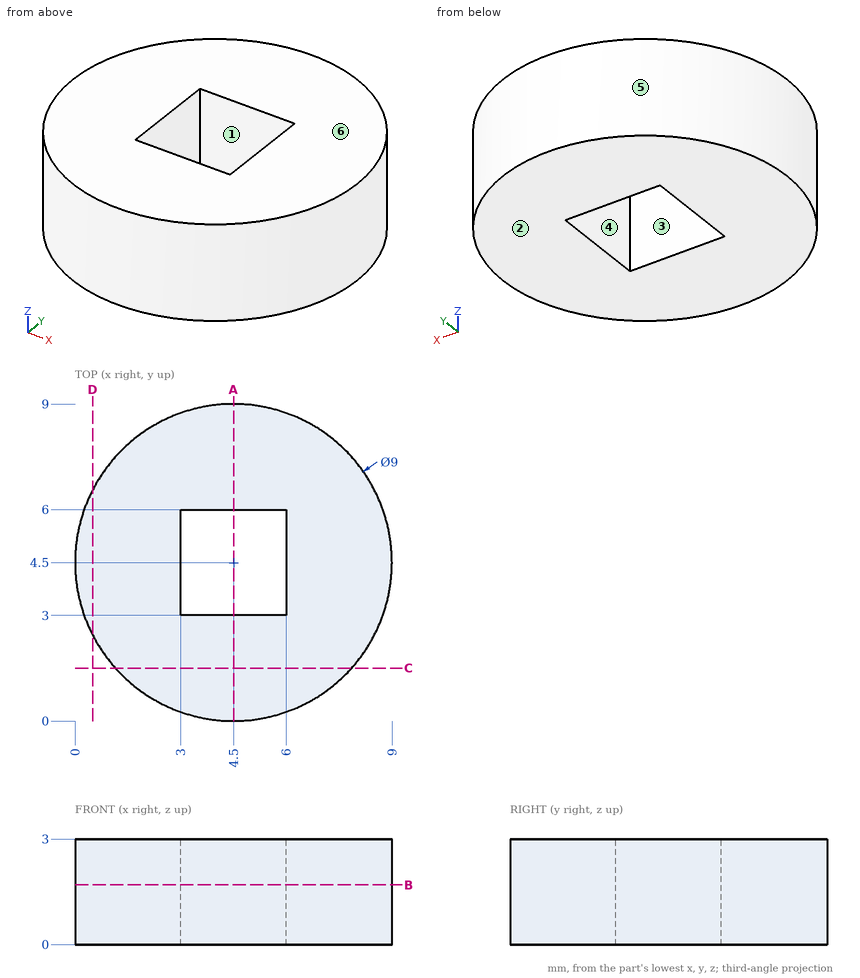
Design review of the part shown in the three views and the two pictorial views. Dimensions are in mm from the part's minimum x, y and z. A direction names the side the tool comes from. Give positions to 0.01 mm unless a question says otherwise; leave off trailing zeros. Write each loop counter-clockwise with the first axis right and the second up, starting at its lowest first coordinate (ties: lowest second). Pieces come first, ordered by that corner, then holes. Notation, with made-up numbers: (80, 42.25) -> (132, 42.25) arc R35 cw to (132, 75.25) -> close; hole circle Ø8 at (-37, -14). An arc over 180 degrees is marked (long way). Answer in a Markdown table with one row per item.
1) Add section C-C on y = 1.5. State the section outline as (x, z) points, plus the area to 3 significant figures.
Worked answers:
| item | result |
|---|---|
| outline | (1.15, 0) -> (7.85, 0) -> (7.85, 3) -> (1.15, 3) -> close |
| area | 20.1 mm² |
2) Add section A-A on x = 4.5. State the section outline as (y, z) points, plus the area to 3 significant figures.
Worked answers:
| item | result |
|---|---|
| outline | (0, 0) -> (3, 0) -> (3, 3) -> (0, 3) -> close; (6, 0) -> (9, 0) -> (9, 3) -> (6, 3) -> close |
| area | 18.0 mm² |
3) Add section D-D on x = 0.5. State the section outline as (y, z) points.
Worked answers:
| item | result |
|---|---|
| outline | (2.44, 0) -> (6.56, 0) -> (6.56, 3) -> (2.44, 3) -> close |
4) For L1, parallel to X at y = 3.25, z = 1.7; L2, parallel to Y at x = 4, z = 0.55; L3, parallel to X at y = 2, z = 1.4, list the stretches that pass through material, from the lowest coordinate up. Write a range as [from, to].
Worked answers:
| item | result |
|---|---|
| L1 | [0.18, 3], [6, 8.82] |
| L2 | [0.03, 3], [6, 8.97] |
| L3 | [0.76, 8.24] |
5) Add section B-B on z = 1.7. State the section outline as (x, y) points, plus the area to 3 significant figures.
Worked answers:
| item | result |
|---|---|
| outline | circle Ø9 at (4.5, 4.5); hole (3, 3) -> (6, 3) -> (6, 6) -> (3, 6) -> close |
| area | 54.6 mm² |
6) Tool access review of the marked faces 1 and 2: name each direction out of +Z, -Z, +X, -X, +Y, -Y from which nothing blocks a thin tool from reaching the whole face with its end or side.
Worked answers:
| item | result |
|---|---|
| face 1 | +Z, -Z |
| face 2 | -Z, +X, -X, +Y, -Y |
7) Mouldability with a two-part tool opening along Y and no side actions: class the marked faces 3, 4, 5 and 6 as +Y half, -Y half, draft (parallel to the pull), parting line (faces both ways), or undercut.
Worked answers:
| item | result |
|---|---|
| face 3 | undercut |
| face 4 | undercut |
| face 5 | parting line |
| face 6 | draft |
